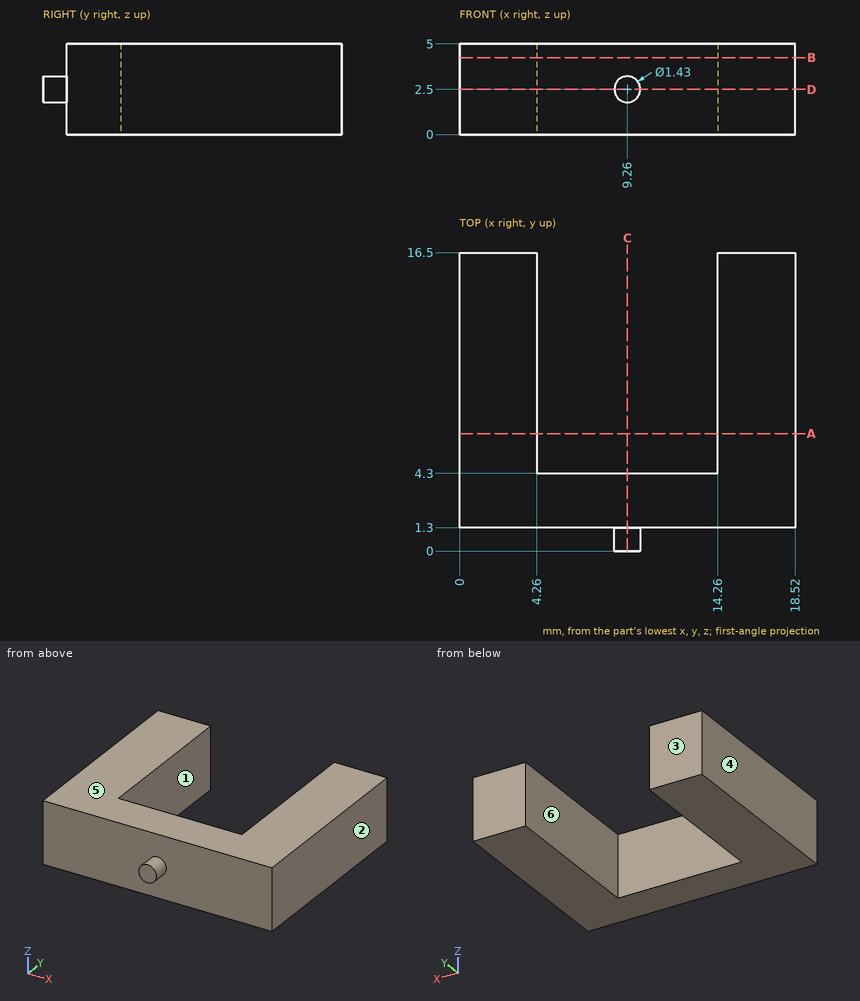
Verification items for this drawing (mm, ordinates from the low corner). A direction names the side the tool comes from. Round coordinates to 2 decimals unless told otherwise and drop trailing zeros. Order: outer loops, then holes, each group sorted by start corner. A loop starts at its lowest first (then second) coordinate and runs counter-clockwise, first axis right, second up. Notation, with made-up numbers: (50, -31.75) - (86, -31.75) arc R26 ccw to (86, -10.75) - close; hole circle Ø8 at (58, 74.5). An arc over 180 degrees is marked (long way). Answer as CSV lines item,"result". Start each with the question number.
1) Tool access check on the marked faces 5 and 6. Record the directions out of +Z, -Z, +X, -X, +Y, -Y that give a thin tool (end or side, any length) a straight path to the whole face; none if there is none.
2) Section check C-C (x = 9.26). Record the cut outline in (y, z) (3 decimals).
3) Depth check by flat-ended pin: pin 1 (1.5 mm diameter, centred on x = 10, z = 3.5, fed in from +Y). Enter the tip coordinate at first touch or a pass-through.
4) Section check A-A (y = 6.5). Record the cut outline in (x, z).
5) Section check D-D (z = 2.5). Record the cut outline in (x, y) (3 decimals), then the cut area to 3 significant figures.
6) Draft check along X on the marked faces 1, 2, 3 and 4. Enter one of: +X half, -X half, draft (parallel to the pull), parting line (faces both ways), or undercut.
7) Scan lines: probe 1 along X at (y, z) = (12.75, 4.8); probe 2 along Y at (x, z) = (6.25, 2.75); probe 3 along Y at (x, z) = (15.5, 2.2). Record each from-to range of solid material in increasing order.
8) Section check B-B (z = 4.25). Record the cut outline in (x, y).
Determined:
1,face 5,"+Z, +X, -X, +Y, -Y"
1,face 6,"+Z, -Z, +Y"
2,outline,"(0, 1.785) - (1.3, 1.785) - (1.3, 0) - (4.3, 0) - (4.3, 5) - (1.3, 5) - (1.3, 3.215) - (0, 3.215) - close"
3,pin 1,"y = 4.3"
4,outline,"(0, 0) - (4.26, 0) - (4.26, 5) - (0, 5) - close; (14.26, 0) - (18.52, 0) - (18.52, 5) - (14.26, 5) - close"
5,outline,"(0, 1.3) - (8.545, 1.3) - (8.545, 0) - (9.975, 0) - (9.975, 1.3) - (18.52, 1.3) - (18.52, 16.5) - (14.26, 16.5) - (14.26, 4.3) - (4.26, 4.3) - (4.26, 16.5) - (0, 16.5) - close"
5,area,"161 mm^2"
6,face 1,"undercut"
6,face 2,"+X half"
6,face 3,"draft"
6,face 4,"-X half"
7,probe 1,"0 to 4.26, 14.26 to 18.52"
7,probe 2,"1.3 to 4.3"
7,probe 3,"1.3 to 16.5"
8,outline,"(0, 1.3) - (18.52, 1.3) - (18.52, 16.5) - (14.26, 16.5) - (14.26, 4.3) - (4.26, 4.3) - (4.26, 16.5) - (0, 16.5) - close"
